Can you work these out from the model? Positions are in its coordinate system, mm. A direction names the side the tool comes from. Round coordinates to 2 decimals unless told otherwise and drop trailing zeros. Loops run counter-clockwise (first coordinate to the right, second up) from the corner with the lowest first, then second, coordinate; pieces in that order, holes last. Notation, with made-up numbers: (63, 1) -> (105, 1) arc R17 ccw to (105, 29) -> close; hole circle Ø11 at (2.25, 20). An arc over 180 degrees is marked (long way). Use a Markdown table: item, result.
from build123d import *

# Parameters (mm, degrees)
SKETCH_W        = 104
SKETCH_H        = 44
PAD_DEPTH       = 20
SKETCH001_W     = 100
SKETCH001_H     = 40
POCKET_DEPTH    = 17
SKETCH002_W     = 68.5
SKETCH002_H     = 30.7
POCKET001_DEPTH = 3
SKETCH003_R     = 1
POCKET002_DEPTH = 2


with BuildPart() as part:
    # Sketch → Pad (new body)
    with BuildSketch(Plane.XY):
        Rectangle(SKETCH_W, SKETCH_H)
    extrude(amount=PAD_DEPTH)

    # Sketch001 (on Face6 of Pad) → Pocket (cut)
    with BuildSketch(Plane.XY.offset(20)):
        Rectangle(SKETCH001_W, SKETCH001_H)
    extrude(amount=-POCKET_DEPTH, mode=Mode.SUBTRACT)

    # Sketch002 (on Face11 of Pocket) → Pocket001 (cut)
    with BuildSketch(Plane.XY.offset(3)):
        Rectangle(SKETCH002_W, SKETCH002_H)
    extrude(amount=-POCKET001_DEPTH, mode=Mode.SUBTRACT)

    # Sketch003 (on Face15 of Pocket001) → Pocket002 (cut)
    with BuildSketch(Plane.XY.offset(3)):
        with Locations((47.5, 17.5)):
            Circle(SKETCH003_R)
        with Locations((-47.5, -17.5)):
            Circle(SKETCH003_R)
    extrude(amount=-POCKET002_DEPTH, mode=Mode.SUBTRACT)


solid = part.part
1. I want a section at B-B (x = 25). Please give me the cut outline in (y, z).
Answer sheet:
| item | result |
|---|---|
| outline | (-22, 0) -> (-15.35, 0) -> (-15.35, 3) -> (-20, 3) -> (-20, 20) -> (-22, 20) -> close; (15.35, 0) -> (22, 0) -> (22, 20) -> (20, 20) -> (20, 3) -> (15.35, 3) -> close |
2. Which directions (+Z, -Z, +X, -X, +Y, -Y) give clear straight access to the entire face, cutting with the end or side of a thin tool? Please do faces 1 (the flat face through (-1, -22, 10)), 2 (the flat face through (-34.25, 0, 2)), 3 (the flat face through (-50, 0, 12)).
Answer sheet:
| item | result |
|---|---|
| face 1 | +Z, -Z, +X, -X, -Y |
| face 2 | +Z, -Z |
| face 3 | +Z |
3. If we mould it in two halves opening along X, with no side actions, what happens to faces 4 (the flat face through (-12, -19, 0)), 5 (the cylindrical face through (-47.04, -18.39, 2.01)), 6 (the flat face through (47, 18, 1)), 7 (the flat face through (52, 0, 10))? For each: +X half, -X half, draft (parallel to the pull), parting line (faces both ways), or undercut.
Answer sheet:
| item | result |
|---|---|
| face 4 | draft |
| face 5 | undercut |
| face 6 | undercut |
| face 7 | +X half |
4. I want a section at C-C (y = -7). Please give me the cut outline in (x, z).
Answer sheet:
| item | result |
|---|---|
| outline | (-52, 0) -> (-34.25, 0) -> (-34.25, 3) -> (-50, 3) -> (-50, 20) -> (-52, 20) -> close; (34.25, 0) -> (52, 0) -> (52, 20) -> (50, 20) -> (50, 3) -> (34.25, 3) -> close |
5. I want a section at D-D (x = 35.5). Please give me the cut outline in (y, z), plus the area to 3 significant figures.
Answer sheet:
| item | result |
|---|---|
| outline | (-22, 0) -> (22, 0) -> (22, 20) -> (20, 20) -> (20, 3) -> (-20, 3) -> (-20, 20) -> (-22, 20) -> close |
| area | 200 mm² |
6. I want a section at A-A (z = 10.75). Please give me the cut outline in (x, y), plus the area to 3 significant figures.
Answer sheet:
| item | result |
|---|---|
| outline | (-52, -22) -> (52, -22) -> (52, 22) -> (-52, 22) -> close; hole (-50, -20) -> (50, -20) -> (50, 20) -> (-50, 20) -> close |
| area | 576 mm² |
7. I need wall thicknesses on line 1 (Y direction, x = 47.5, z = 2.2); line 2 (Y direction, x = -44.5, z = 12); line 3 (X direction, y = -6, z = 3.25). Which ranges of each line are inside material? Lowest first, please.
Answer sheet:
| item | result |
|---|---|
| line 1 | y = -22 to 16.5, 18.5 to 22 |
| line 2 | y = -22 to -20, 20 to 22 |
| line 3 | x = -52 to -50, 50 to 52 |
8. Will these pins go through, and if not, where does the flat tip stop? pin 1 Ø1.8 at (x, y) = (-47.5, -17.5) entering from +Z; pin 2 Ø10 at (x, y) = (-31, 10) entering from +Z.
Answer sheet:
| item | result |
|---|---|
| pin 1 | stops at z = 1 |
| pin 2 | stops at z = 3 |
